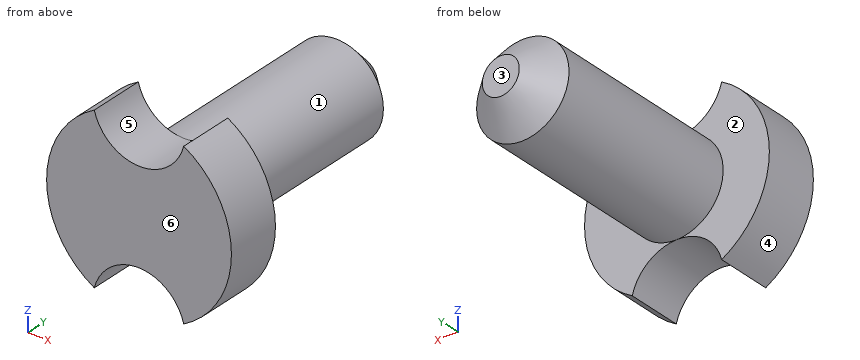
Autodesk Inventor part; units mm, degrees
ref_plane "YZ Plane" through (0, 0, 0) normal (1, 0, 0) x (0, 1, 0)
ref_plane "XZ Plane" through (0, 0, 0) normal (0, 1, 0) x (-1, 0, 0)
ref_plane "XY Plane" through (0, 0, 0) normal (0, 0, 1) x (1, 0, 0)
sketch "Sketch1" plane through (0, 0, 0) normal (0, 1, 0) x (-1, 0, 0)
  circle A0 centre (0, 0) radius 2.5
  circle A1 centre (0, 2.5) radius 1.25
  circle A2 centre (0, -2.5) radius 1.25
  point P0 (-1.2103, -2.1875)
  point P1 (1.2103, -2.1875)
  point P2 (1.2103, 2.1875)
  point P3 (-1.2103, 2.1875)
  dimension "d0" = 5
  dimension "d1" = 2.5
  dimension "d2" = 2.5
extrude "Extrusion1" add sketch "Sketch1" along normal blind 1.5 contours A0 A2 A1
sketch "Sketch2" plane through (0, 1.5, 0) normal (0, 1, 0) x (1, 0, 0)
  circle A0 centre (0, 0) radius 1.25
  dimension "d5" = 2.5
extrude "Extrusion2" add sketch "Sketch2" along normal blind 6
chamfer "Chamfer1" distance 0.75 angle 45 1 edges at (-1.25, 7.5, 0)
properties part number "hot_pin_6"
The model under review builds one solid part; all positions refer to its coordinate system, in mm. Face numbers are marked on the shaded views. A direction names the side the tool comes from. Round coordinates to 2 decimals unless told otherwise and drop trailing zeros. Loops run counter-clockwise (first coordinate to the right, second up) from the corner with the lowest first, then second, coordinate; pieces in that order, holes last. Notation, with made-up numbers: (-38, 46.25) -> (20, 46.25) arc R24 cw to (20, 67.25) -> close; hole circle Ø5 at (-13.5, 81). An arc over 180 degrees is marked (long way). Return JSON: item names as keys, results as strings.
(1) Add section B-B on z = 0. Write out the cut boundary in (x, y), plus the area to 3 significant figures.
Solved:
{"outline": "(-2.5, 0) -> (2.5, 0) -> (2.5, 1.5) -> (1.25, 1.5) -> (1.25, 6.75) -> (0.5, 7.5) -> (-0.5, 7.5) -> (-1.25, 6.75) -> (-1.25, 1.5) -> (-2.5, 1.5) -> close", "area": "21.9 mm2"}
(2) For line 1 (Y direction, x = -1.7, z = 0.7); line 2 (Z direction, x = 0.2, y = 2.25); line 3 (X direction, y = 4.5, z = -0.75), list the stretches that pass through material, from the lowest coordinate up.
Solved:
{"line 1": "0 to 1.5", "line 2": "-1.23 to 1.23", "line 3": "-1 to 1"}
(3) Add section C-C on y = 3.5. Write out the cut boundary in (x, z).
Solved:
{"outline": "circle Ø2.5 at (0, 0)"}
(4) Add section A-A on z = 1.7. Write out the cut boundary in (x, y), plus the area to 3 significant figures.
Solved:
{"outline": "(-1.83, 0) -> (-0.96, 0) -> (-0.96, 1.5) -> (-1.83, 1.5) -> close; (0.96, 0) -> (1.83, 0) -> (1.83, 1.5) -> (0.96, 1.5) -> close", "area": "2.62 mm2"}
(5) For the marked faces 1, 2 and 3, list the 3-axis set-ups (+Z, -Z, +X, -X, +Y, -Y) from which the entire face can be reached by the end or side of a thin tool; tool diameter is ignored.
Solved:
{"face 1": "+Y", "face 2": "-X, +Y", "face 3": "+Z, -Z, +X, -X, +Y"}
(6) The part is to be moulded in two halves that separate along X. For the marked faces 4, 5 and 6, say which applies: released by +X, released by -X, zero draft, split by the parting line, or undercut.
Solved:
{"face 4": "released by -X", "face 5": "undercut", "face 6": "zero draft"}
(7) For pin 1 (2 mm diameter, centred on x = -2, z = 0.5, fed in from +Y); pin 2 (1.5 mm diameter, centred on y = 4, z = 0.5, fed in from -X); pin 3 (1.5 mm diameter, centred on x = -0.5, z = -1.5, fed in from +Y), all flat-tipped, find the tip position at first contact; note any pin that passes through.
Solved:
{"pin 1": "y = 6.94", "pin 2": "x = -1.25", "pin 3": "y = 7.17"}
(8) Add section D-D on x = -1.55. Write out the cut boundary in (y, z), plus the area to 3 significant figures.
Solved:
{"outline": "(0, -1.96) -> (1.5, -1.96) -> (1.5, 1.96) -> (0, 1.96) -> close", "area": "5.88 mm2"}
